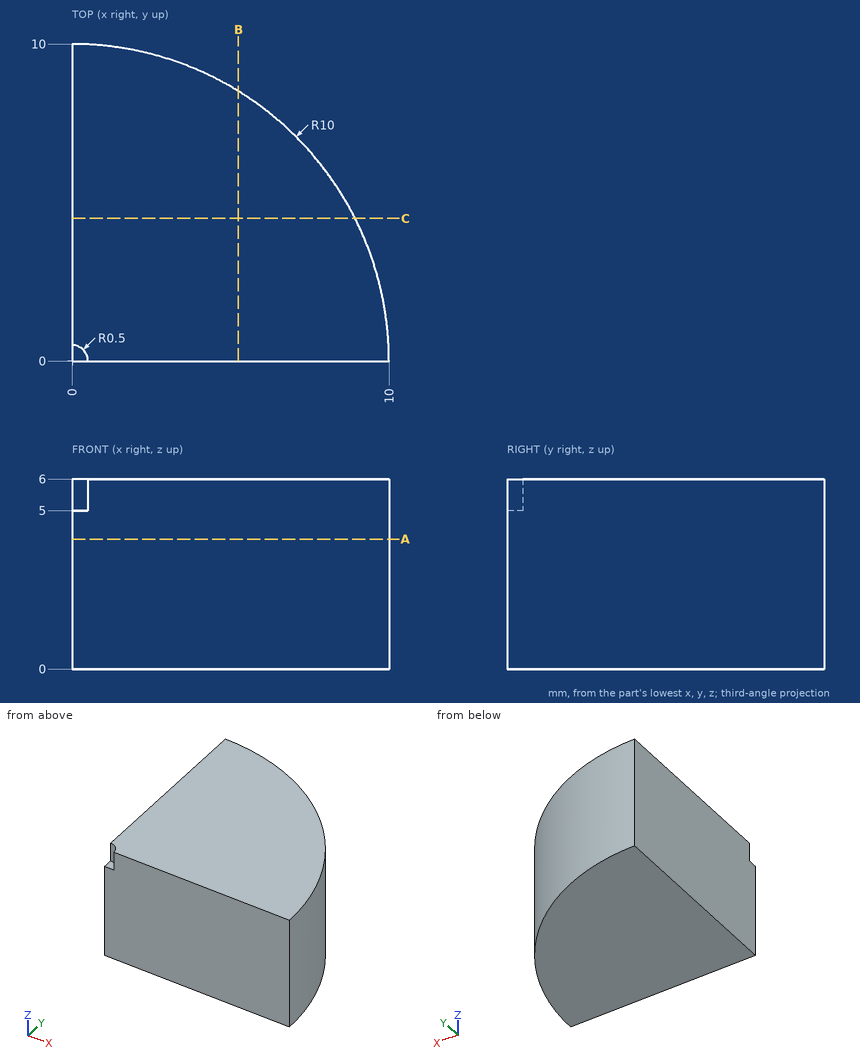
The drawing under review shows one solid part. Ordinate dimensions are in mm from its lowest x, y, z. Round coordinates to 2 decimals unless told otherwise and drop trailing zeros. Write each loop counter-clockwise with the first axis right and the second up, starting at its lowest first coordinate (ties: lowest second). Pieces come first, ordered by that corner, then holes.
(1) We need section A-A on z = 4.1. Give the boundary of the cut face in (x, y), and give its area (3 significant figures).
(2) We need section C-C on y = 4.5. Give the boundary of the cut face in (x, z), and give its area (3 significant figures).
(3) Wall thickness on L1, parallel to X at y = 8, z = 1.55; L2, parallel to X at y = 9, z = 2.95; L3, parallel to Y at x = 5.25, z = 3: over which ranges is each line inside the solid? List them lowest first.
(4) We need section B-B on x = 5.25. Give the boundary of the cut face in (y, z).
(5) Insertion check: pin 1 (3 mm diameter, centred on y = 8, z = 1, fed in from +X); pin 2 (1.5 mm diameter, centred on x = 8.5, z = 3.5, fed in from +Y); pin 3 (3 mm diameter, centred on y = 8.5, z = 4.5, fed in from +X). Each pin has a flat end and moves straight along its axis. Give the tip position at first contact, or say it passes through.
Findings below:
1. outline: (0, 0) - (10, 0) arc R10 ccw to (0, 10) - close
1. area: 78.5 mm2
2. outline: (0, 0) - (8.93, 0) - (8.93, 6) - (0, 6) - close
2. area: 53.6 mm2
3. L1: x = 0 to 6
3. L2: x = 0 to 4.36
3. L3: y = 0 to 8.51
4. outline: (0, 0) - (8.51, 0) - (8.51, 6) - (0, 6) - close
5. pin 1: stops at x = 7.6
5. pin 2: stops at y = 6.32
5. pin 3: stops at x = 7.14
